Read the model definition and answer for the solid it produces. Units are mm, in the model's axes. Coordinates: 2 decimals unless noted, no trailing zeros. Write each loop counter-clockwise with the first axis right and the second up, starting at its lowest first coordinate (ties: lowest second). Pieces come first, ordered by that corner, then holes. Notation, with made-up numbers: (-35.5, -24) - (-22.5, -24) arc R11 ccw to (-22.5, -8) - close; hole circle Ø4 at (-17, 38). An arc over 180 degrees is marked (long way). Use a Markdown table: item, result.
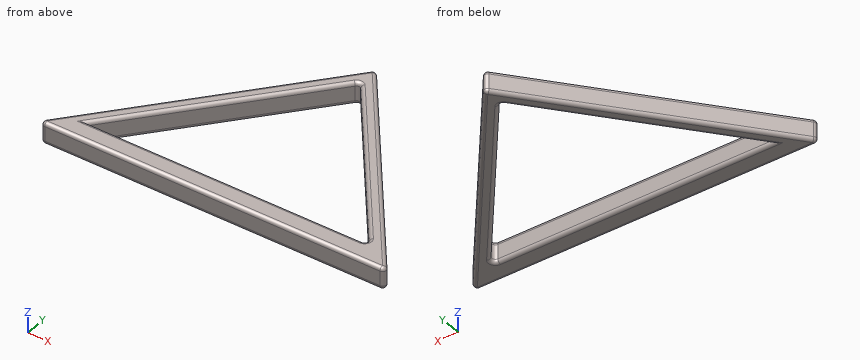
from build123d import *

# Parameters (mm, degrees)
F1_DEPTH = 30
F2_R     = 5


with BuildPart() as f1:
    # F0 (on Top) → F1 (new body)
    with BuildSketch(Plane.XY):
        Polygon((-248, -30), (0, -30), (248, -30), (0, 280), align=None)
        Polygon((200, 0), (0, 0), (-200, 0), (0, 250), align=None, mode=Mode.SUBTRACT)
    extrude(amount=F1_DEPTH)

    # F2
    f2_edges = [f1.edges().sort_by_distance(p)[0] for p in [
        (0, 280, 15),
        (-248, -30, 15),
        (-124, 125, 0),
        (-124, 125, 30),
        (248, -30, 15),
        (124, 125, 0),
        (124, 125, 30),
        (0, -30, 30),
        (0, -30, 0),
        (0, 0, 30),
        (-100, 125, 30),
        (0, 250, 15),
        (200, 0, 15),
        (100, 125, 0),
        (100, 125, 30),
        (0, 0, 0),
        (-100, 125, 0),
    ]]
    fillet(f2_edges, radius=F2_R)


solid = f1.part
(1) Straight lines are drawn through the part: L1, parallel to X at y = 101.5, z = 8.5; L2, parallel to Y at x = 189, z = 9.5; L3, parallel to Y at x = 181, z = 9.5. For each, find the intervals that lie inside material, in ascending order.
Report:
| item | result |
|---|---|
| L1 | x = -142.8 to -118.8, 118.8 to 142.8 |
| L2 | y = -30 to 0, 13.75 to 43.75 |
| L3 | y = -30 to 0, 23.75 to 53.75 |
(2) Each of these flat-tipped pins is pushed along its axis until it touches: P1, Ø1.5, axis at y = 207.5, z = 19, coming from the +X side; P2, Ø8, axis at x = -107.5, y = 146.5, coming from the +Z side; P3, Ø4, axis at y = 39, z = 27, coming from the +X side. Where does it stop, or does it pass through?
Report:
| item | result |
|---|---|
| P1 | stops at x = 58.6 |
| P2 | stops at z = 29.75 |
| P3 | stops at x = 194.08 |
(3) A cutting plane is placed at A-A, the plane z = 17.5. Write down the section's boundary in (x, y).
Report:
| item | result |
|---|---|
| outline | (-241.5, -21.88) arc R5 ccw to (-237.6, -30) - (237.6, -30) arc R5 ccw to (241.5, -21.88) - (3.9, 275.12) arc R5 ccw to (-3.9, 275.12) - close; hole (-200, 0) - (189.6, 0) arc R5 ccw to (193.5, 8.12) - (3.9, 245.12) arc R5 ccw to (-3.9, 245.12) - close |
